Can you work these out from the model? Positions are in its coordinate system, mm. Face numbers are marked on the shaded views. A direction names the side the tool comes from. Give positions to 0.01 mm unless a question says otherwise; leave off trailing zeros. Write each loop counter-clockwise with the first axis right and the second up, starting at its lowest first coordinate (ties: lowest second). Pieces come first, ordered by that corner, then holes. Notation, with made-up numbers: (26, 28.5) - (67, 28.5) arc R20 ccw to (67, 47.5) - close; hole circle Ø9 at (-18, 48.25). An arc over 180 degrees is marked (long way). Use a Markdown table: item, result. Add a question column.
```python
from build123d import *

# Parameters (mm, degrees)
SKETCH1_W                = 40
SKETCH1_H                = 40
SKETCH1_W_2              = 20
SKETCH1_H_2              = 20
BOSS_EXTRUDE1_DEPTH      = 105.5
SKETCH2_W                = 102.5
SKETCH2_H                = 100
SKETCH2_W_2              = 82.5
SKETCH2_H_2              = 80
BOSS_EXTRUDE2_DEPTH      = 100
EXTRUDE_THIN1_DEPTH      = 158
EXTRUDE_THIN1_DEPTH_BACK = 166
RIB8_START               = -2.5
RIB8_DEPTH               = 5
CUT_EXTRUDE2_DEPTH       = 338.270292199
SKETCH2_2_W              = 82.5
SKETCH2_2_H              = 80
CUT_EXTRUDE3_DEPTH       = 299.029885246
SKETCH1_2_W              = 20
SKETCH1_2_H              = 20
CUT_EXTRUDE4_DEPTH       = 299.029885246
BOSS_EXTRUDE3_REACH      = 300.03
SKETCH7_R                = 5
BOSS_EXTRUDE4_REACH      = 300.03
CUT_EXTRUDE6_DEPTH       = 299.029885246
CUT_EXTRUDE6_DEPTH_BACK  = 299.029885246
SKETCH7_4_R              = 5
BOSS_EXTRUDE5_DEPTH      = 14


# Read off the part's stored shape, not the designer's step: Rib8
with BuildPart() as part:
    # Sketch1 → Boss-Extrude1 (new body)
    with BuildSketch(Plane.XY):
        Rectangle(SKETCH1_W, SKETCH1_H)
        Rectangle(SKETCH1_W_2, SKETCH1_H_2, mode=Mode.SUBTRACT)
    extrude(amount=BOSS_EXTRUDE1_DEPTH)



with BuildPart() as body_2:
    # Sketch2 → Boss-Extrude2 (new body)
    with BuildSketch(Plane.XY.offset(145.5)):
        with Locations((0, -205)):
            Rectangle(SKETCH2_W, SKETCH2_H)
        with Locations((0, -205)):
            Rectangle(SKETCH2_W_2, SKETCH2_H_2, mode=Mode.SUBTRACT)
    extrude(amount=-BOSS_EXTRUDE2_DEPTH)


with BuildPart() as part_1:
    add(part.part)

    add(body_2.part)  # Extrude-Thin1 merges body 2
    # Sketch3 → Extrude-Thin1 (add, two sides: drawn at the far end of the back side and taken through both)
    with BuildSketch(Plane(origin=(0, 0, 0), x_dir=(0, 0, -1), z_dir=(1, 0, 0)).offset(-EXTRUDE_THIN1_DEPTH_BACK)):
        Polygon((-105.5, 20), (-105.5, 0), (-105.5, -60), (-145.5, -93.563985247), (-145.5, -255), (-139.5, -255), (-139.5, -96.361831196), (-99.5, -62.797845949), (-99.5, 0), (-99.5, 20), align=None)
    extrude(amount=EXTRUDE_THIN1_DEPTH + EXTRUDE_THIN1_DEPTH_BACK)

    # Rib8 outline → Rib8 (add)
    with BuildSketch(Plane.YZ.offset(RIB8_START)):
        Polygon((-38.377112489, 0), (-20, 0), (-20, 99.5), (-62.797845949, 99.5), (-96.361831196, 139.5), (-155, 139.5), (-155, 45.5), (-76.556145708, 45.5), align=None)
    extrude(amount=RIB8_DEPTH)

    # Sketch6 → Cut-Extrude2 (cut, through all)
    with BuildSketch(Plane.XY.offset(145.5)):
        Polygon((20, 20), (20, 0), (51.25, -199), (51.25, -255), (158, -255), (158, 20), align=None)
        Polygon((-51.25, -255), (-158, -255), (-166, -255), (-166, 20), (-158, 20), (-20, 20), (-20, 0), (-51.25, -199), align=None)
    extrude(amount=-CUT_EXTRUDE2_DEPTH, mode=Mode.SUBTRACT)

    # Sketch2<2> → Cut-Extrude3 (cut, through all)
    with BuildSketch(Plane.XY.offset(145.5)):
        with Locations((0, -205)):
            Rectangle(SKETCH2_2_W, SKETCH2_2_H)
    extrude(amount=-CUT_EXTRUDE3_DEPTH, mode=Mode.SUBTRACT)

    # Sketch1<2> → Cut-Extrude4 (cut, through all)
    with BuildSketch(Plane.XY):
        Rectangle(SKETCH1_2_W, SKETCH1_2_H)
    extrude(amount=CUT_EXTRUDE4_DEPTH, mode=Mode.SUBTRACT)

    # Boss-Extrude3: up to this plane
    boss_extrude3_end = Plane(origin=(-20, 0, 0), z_dir=(-0.9878934335848292, 0.15513401909309493, 0))
    # Sketch7 → Boss-Extrude3 (add, up to the surface)
    with BuildSketch(Plane(origin=(0, 0, 0), x_dir=(0, 0, -1), z_dir=(1, 0, 0)), mode=Mode.PRIVATE) as boss_extrude3_sk1:
        with BuildLine():
            Line((-145.5, -165), (-125.5, -165))
            Line((-125.5, -165), (-125.5, -140))
            ThreePointArc((-125.5, -140), (-128.428932188, -132.928932188), (-135.5, -130))
            Line((-135.5, -130), (-145.5, -130))
            Line((-145.5, -130), (-145.5, -165))
        make_face()
        with Locations((-135.5, -140)):
            Circle(SKETCH7_R, mode=Mode.SUBTRACT)
    boss_extrude3_tool1 = split(extrude(boss_extrude3_sk1.sketch, amount=-BOSS_EXTRUDE3_REACH, mode=Mode.PRIVATE), bisect_by=boss_extrude3_end, keep=Keep.BOTH, mode=Mode.PRIVATE)
    add(boss_extrude3_tool1.solids().sort_by_distance((0, -149.027778, 135.777778))[0])
    # Sketch7 → Boss-Extrude3 (add, up to the surface)
    with BuildSketch(Plane(origin=(0, 0, 0), x_dir=(0, 0, -1), z_dir=(1, 0, 0)), mode=Mode.PRIVATE) as boss_extrude3_sk2:
        with BuildLine():
            Line((-105.5, -10), (-85.5, -10))
            Line((-85.5, -10), (-85.5, -30))
            ThreePointArc((-85.5, -30), (-88.428932188, -37.071067812), (-95.5, -40))
            Line((-95.5, -40), (-105.5, -40))
            Line((-105.5, -40), (-105.5, -10))
        make_face()
        with Locations((-95.5, -30)):
            Circle(SKETCH7_R, mode=Mode.SUBTRACT)
    boss_extrude3_tool2 = split(extrude(boss_extrude3_sk2.sketch, amount=-BOSS_EXTRUDE3_REACH, mode=Mode.PRIVATE), bisect_by=boss_extrude3_end, keep=Keep.BOTH, mode=Mode.PRIVATE)
    add(boss_extrude3_tool2.solids().sort_by_distance((0, -23.666667, 95.833333))[0])

    # Boss-Extrude4: up to this plane
    boss_extrude4_end = Plane(origin=(20, 0, 0), z_dir=(-0.9878934335848292, -0.15513401909309524, 0))
    # Sketch7<2> → Boss-Extrude4 (add, up to the surface)
    with BuildSketch(Plane(origin=(0, 0, 0), x_dir=(0, 0, -1), z_dir=(1, 0, 0)), mode=Mode.PRIVATE) as boss_extrude4_sk1:
        with BuildLine():
            Line((-145.5, -165), (-125.5, -165))
            Line((-125.5, -165), (-125.5, -140))
            ThreePointArc((-125.5, -140), (-128.428932188, -132.928932188), (-135.5, -130))
            Line((-135.5, -130), (-145.5, -130))
            Line((-145.5, -130), (-145.5, -165))
        make_face()
    boss_extrude4_tool1 = split(extrude(boss_extrude4_sk1.sketch, amount=BOSS_EXTRUDE4_REACH, mode=Mode.PRIVATE), bisect_by=boss_extrude4_end, keep=Keep.BOTH, mode=Mode.PRIVATE)
    add(boss_extrude4_tool1.solids().sort_by_distance((0, -147.982828, 135.745625))[0])
    # Sketch7<2> → Boss-Extrude4 (add, up to the surface)
    with BuildSketch(Plane(origin=(0, 0, 0), x_dir=(0, 0, -1), z_dir=(1, 0, 0)), mode=Mode.PRIVATE) as boss_extrude4_sk2:
        with BuildLine():
            Line((-105.5, -10), (-85.5, -10))
            Line((-85.5, -10), (-85.5, -30))
            ThreePointArc((-85.5, -30), (-88.428932188, -37.071067812), (-95.5, -40))
            Line((-95.5, -40), (-105.5, -40))
            Line((-105.5, -40), (-105.5, -10))
        make_face()
    boss_extrude4_tool2 = split(extrude(boss_extrude4_sk2.sketch, amount=BOSS_EXTRUDE4_REACH, mode=Mode.PRIVATE), bisect_by=boss_extrude4_end, keep=Keep.BOTH, mode=Mode.PRIVATE)
    add(boss_extrude4_tool2.solids().sort_by_distance((0, -24.52645, 95.788082))[0])

    # Sketch7<4> → Cut-Extrude6 (cut, two sides: drawn at the far end of the back side and taken through both)
    with BuildSketch(Plane(origin=(0, 0, 0), x_dir=(0, 0, -1), z_dir=(1, 0, 0)).offset(-CUT_EXTRUDE6_DEPTH_BACK)):
        with Locations(Location((-135.5, -140, 0), (0, 0, 90))):
            Circle(SKETCH7_4_R)
        with Locations(Location((-95.5, -30, 0), (0, 0, 90))):
            Circle(SKETCH7_4_R)
    extrude(amount=CUT_EXTRUDE6_DEPTH + CUT_EXTRUDE6_DEPTH_BACK, mode=Mode.SUBTRACT)

    # Sketch8 → Boss-Extrude5 (add)
    with BuildSketch(Plane(origin=(0, 0, 99.5), x_dir=(-1, 0, 0), z_dir=(0, 0, -1))):
        Polygon((20, 0), (20, -10), (21.570351759, -10), align=None)
        Polygon((-20, 0), (-21.570351759, -10), (-20, -10), align=None)
    extrude(amount=BOSS_EXTRUDE5_DEPTH)


solid = part_1.part
```
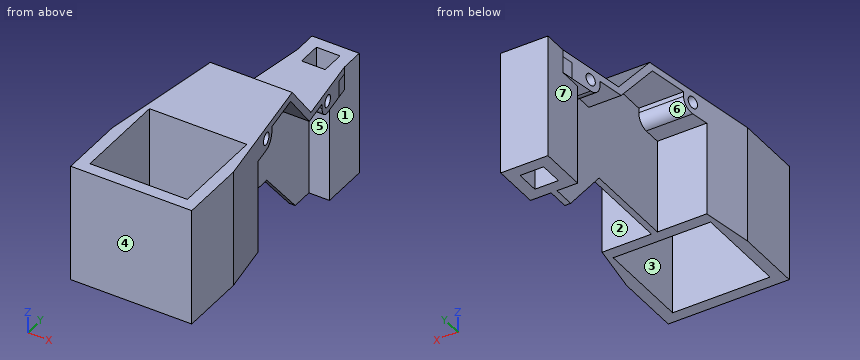
Q1. Suppose I cut it at B-B (z = 79). Please give me the cut outline in (x, y).
Q2. If I drill on probe 1 along Y at (x, z) = (7, 95.5); probe 2 along Y at (x, z) = (26.5, 54); probe 3 along Y at (x, z) = (3, 50), over which ranges is the centre line in solid material (lowest first)? Write a range as [from, to].
Q3. Suppose I cut it at C-C (y = -184.5). Please give me the cut outline in (x, z), and give its area (3 significant figures).
Q4. Suppose I cut it at D-D (z = 38.5). Please give me the cut outline in (x, y), and give its area (3 significant figures).
Q5. If we mould it in two halves opening along Y, with no side actions, what happens to the marked faces 4, 5, 6 and 7? For each: released by +Y, released by -Y, zero draft, split by the parting line, or undercut.
Q6. Suppose I cut it at A-A (x = 17). Please give me the cut outline in (y, z).
Q7. I'm going to push flat-ended pins straight in: P1, Ø2, axis at x = 27, y = -69.5, coming from the -Z side; P2, Ø4.5, axis at x = 14, y = -149, coming from the -Z side; P3, Ø5, axis at x = -13.5, z = 27, coming from the -Y side. Where does each tip first touch, or does it pass through?
Q8. On a 3-axis mill with a long thin cutter (end or side, diameter ignored), from which of +Z, -Z, +X, -X, +Y, -Y can I reach the whole of each face in a straight line? I mean the marked faces 1, 2 and 3. Say none if no direction works.
Derived:
| question | item | result |
|---|---|---|
| 1 | outline | (-51.25, -255) - (51.25, -255) - (51.25, -199) - (44.34, -155) - (2.5, -155) - (2.5, -20) - (20, -20) - (20, 20) - (-20, 20) - (-20, -20) - (-2.5, -20) - (-2.5, -155) - (-44.34, -155) - (-51.25, -199) - close; hole (-41.25, -245) - (41.25, -245) - (41.25, -165) - (-41.25, -165) - close; hole (-10, -10) - (10, -10) - (10, 10) - (-10, 10) - close |
| 2 | probe 1 | [-255, -245], [-165, -155], [-40, -35], [-25, -10], [10, 20] |
| 2 | probe 2 | [-255, -245], [-165, -155] |
| 2 | probe 3 | [-255, -245], [-165, -155], [-20, -10], [10, 20] |
| 3 | outline | (-48.97, 45.5) - (-41.25, 45.5) - (-41.25, 145.5) - (-48.97, 145.5) - close; (41.25, 45.5) - (48.97, 45.5) - (48.97, 145.5) - (41.25, 145.5) - close |
| 3 | area | 1,540 mm² |
| 4 | outline | (-20, -20) - (-2.5, -20) - (-2.5, -70.68) - (2.5, -70.68) - (2.5, -20) - (20, -20) - (20, 20) - (-20, 20) - close; hole (-10, -10) - (10, -10) - (10, 10) - (-10, 10) - close |
| 4 | area | 1,450 mm² |
| 5 | face 4 | released by -Y |
| 5 | face 5 | undercut |
| 5 | face 6 | undercut |
| 5 | face 7 | zero draft |
| 6 | outline | (-255, 45.5) - (-245, 45.5) - (-245, 145.5) - (-255, 145.5) - close; (-165, 45.5) - (-155, 45.5) - (-155, 125.5) - (-140, 125.5) arc R10 ccw to (-130, 135.5) - (-130, 139.5) - (-96.36, 139.5) - (-62.8, 99.5) - (-40, 99.5) - (-40, 95.5) arc R10 ccw to (-30, 85.5) - (-20, 85.5) - (-20, 0) - (20, 0) - (20, 105.5) - (-60, 105.5) - (-93.56, 145.5) - (-165, 145.5) - close; hole circle Ø10 at (-140, 135.5); hole circle Ø10 at (-30, 95.5) |
| 7 | P1 | z = 106.3 |
| 7 | P2 | z = 125.5 |
| 7 | P3 | y = -20 |
| 8 | face 1 | -Z, +X, +Y |
| 8 | face 2 | -Z, +X |
| 8 | face 3 | +Z, -Z |
